Source: CAD feature listing. Evaluate the final solid. Frame: model axes, mm. A direction names the side the tool comes from. Coordinates: 2 decimals unless noted, no trailing zeros. Loops run counter-clockwise (first coordinate to the right, second up) from the corner with the lowest first, then second, coordinate; pieces in that order, holes last.
Item 1: Section query C-C, the plane z = 24. Return the cut outline in (x, y).
Item 2: Reachability of faces 1 (the flat face through (2, -19.812, -8)), 2 (the flat face through (2, 9.688, -8)), 3 (the flat face through (2, 6.888, -22)), 4 (the flat face through (2, 7.688, -22)), 5 (the cylindrical face through (7.73, -3.31, 5.18)) from +Z, -Z, +X, -X, +Y, -Y: full face, straight path, thin tool, end or side. Return the list, or none.
Item 3: Pull-direction query (Y, two-part tool) for faces 6 (the flat face through (2, -7.112, -22)), 7 (the flat face through (-3.853, -5, -8)), 8 (the flat face through (2, -7.912, -22)); classes: +Y half, -Y half, draft (parallel to the pull), parting line (faces both ways), or undercut.
Item 4: Section query A-A, the plane y = 4.25. Return the cut outline in (x, z), then the cut area to 3 significant figures.
Item 5: Section query B-B, the plane y = -9.25. Return the cut outline in (x, z), then the cut area to 3 significant figures.
Item 6: Pin query (flat end, axial travel): pin 1 Ø0.6 at (y, z) = (7.5, -20.5) entering from -X; pin 2 Ø3 at (x, z) = (2, -22.5) entering from -Y; pin 3 Ø3 at (x, y) = (3.5, 3) entering from +Z. Return the tip coordinate at first contact, or that it passes through.
Item 7: Line query: probe 1 along Z at (x, y) = (2, 2.5); probe 2 along Z at (x, y) = (7.75, -6.25); probe 3 along Y at (x, z) = (-0.75, 5). Output: solid intervals per line, ascending.
Item 8: Section query D-D, the plane z = 5. Return the cut outline in (x, y), then the cut area to 3 significant figures.
```python
from build123d import *

# Parameters (mm, degrees)
F0_W     = 12
F0_H     = 29.5
F0_R     = 5.85
F1_DEPTH = 17
F2_DEPTH = 10.5
F3_R     = 2.65
F4_DEPTH = 17.5
F5_R     = 2
F7_DEPTH = 10.5


with BuildPart() as f1:
    # F0 (on Top) → F1 (new body)
    with BuildSketch(Plane.XY):
        with Locations((2.146811, -5.062469)):
            Rectangle(F0_W, F0_H)
        with Locations((2.146811, -5.062469)):
            Circle(F0_R, mode=Mode.SUBTRACT)
        with Locations((2.146811, -5.062469)):
            Circle(F0_R)
    extrude(amount=-F1_DEPTH)

    # F0 (on Top) → F2 (join)
    with BuildSketch(Plane.XY):
        with Locations((2.146811, -5.062469)):
            Circle(F0_R)
    extrude(amount=F2_DEPTH)

    # F3 (on face) → F4 (join)
    with BuildSketch(Plane.XY.offset(10.5)):
        with Locations((2.146811, -5.062469)):
            Circle(F3_R)
    extrude(amount=F4_DEPTH)

    # F5
    f5_edges = [f1.edges().sort_by_distance(p)[0] for p in [
        (-0.503189, -5.062469, 28),
    ]]
    fillet(f5_edges, radius=F5_R)

    # F6 (on face) → F7 (join)
    with BuildSketch(Plane(origin=(0, 0, -17), x_dir=(1, 0, 0), z_dir=(0, 0, -1))):
        Polygon((-0.953189, 7.112469), (2.146811, 7.112469), (5.246811, 7.112469), (5.246811, 7.912469), (-0.953189, 7.912469), align=None)
        Polygon((-0.953189, -7.687531), (2.146811, -7.687531), (5.246811, -7.687531), (5.246811, -6.887531), (-0.953189, -6.887531), align=None)
    extrude(amount=F7_DEPTH)


solid = f1.part
```
Verdict:
1. outline: circle Ø5.3 at (2.15, -5.06)
2. face 1: +Z, -Z, +X, -X, -Y
2. face 2: +Z, -Z, +X, -X, +Y
2. face 3: -Z, +X, -X
2. face 4: -Z, +X, -X, +Y
2. face 5: +Z
3. face 6: undercut
3. face 7: draft
3. face 8: -Y half
4. outline: (-3.85, -17) - (8.15, -17) - (8.15, 0) - (-3.85, 0) - close
4. area: 204 mm2
5. outline: (-3.85, -17) - (8.15, -17) - (8.15, 0) - (6.23, 0) - (6.23, 10.5) - (-1.94, 10.5) - (-1.94, 0) - (-3.85, 0) - close
5. area: 290 mm2
6. pin 1: stops at x = -0.95
6. pin 2: stops at y = -7.91
6. pin 3: stops at z = 0
7. probe 1: z = -17 to 0
7. probe 2: z = -17 to 10.5
7. probe 3: y = -10.14 to 0.02
8. outline: circle Ø11.7 at (2.15, -5.06)
8. area: 108 mm2
